Check sheet for the modelled part. Datum: model origin and axes. Units: mm. A direction names the side the tool comes from. Round coordinates to 2 decimals unless told otherwise and drop trailing zeros. Write each loop counter-clockwise with the first axis right and the second up, starting at its lowest first coordinate (ties: lowest second). Pieces come first, ordered by that corner, then holes. Notation, with made-up numbers: (-4, 24) -> (30, 24) arc R30 ccw to (30, 51) -> close; hole circle Ø10 at (46.5, 42). An arc over 180 degrees is marked (long way). One line per item, written item: value.
Autodesk Inventor part; units mm, degrees
ref_plane "Start plane" through (0, 0, -63.5) normal (0, 0, 1) x (1, 0, 0)
ref_plane "End plane" through (0, 0, 777.875) normal (0, 0, 1) x (1, 0, 0)
ref_plane "Work Plane3" through (0, -454.025, -63.5) normal (0, 0, -1) x (-1, 0, 0)
ref_plane "Start plane" through (0, 0, -63.5) normal (0, 0, 1) x (1, 0, 0)
ref_plane "End plane" through (0, 0, 777.875) normal (0, 0, 1) x (1, 0, 0)
sketch "Sketch" plane through (0, 0, 0) normal (0, 0, 1) x (1, 0, 0)
  line L0 (63.5, 0) -> (0, 0)
  line L1 (0, 0) -> (0, 63.5)
  line L2 (0, 63.5) -> (0.9525, 63.5)
  line L3 (4.7625, 59.69) -> (4.7625, 12.6365)
  line L4 (12.6365, 4.7625) -> (59.69, 4.7625)
  line L5 (63.5, 0.9525) -> (63.5, 0)
  line L6 (0, -11.0414) -> (0, 31.5385) construction
  line L7 (-11.0414, 0) -> (31.5385, 0) construction
  arc A0 (4.7625, 12.6365) -> (12.6365, 4.7625) centre (12.6365, 12.6365) ccw
  arc A1 (4.7625, 59.69) -> (0.9525, 63.5) centre (0.9525, 59.69) ccw
  arc A2 (63.5, 0.9525) -> (59.69, 4.7625) centre (59.69, 0.9525) ccw
  line L8 (0, 79.3552) -> (0, -26.1075) construction
  line L9 (-26.1075, 0) -> (79.3552, 0) construction
  point P0 (4.7625, 63.5)
  point P1 (4.7625, 4.7625)
  point P2 (63.5, 4.7625)
  dimension "d0" = 63.5
  dimension "d1" = 63.5
  dimension "d2" = 4.7625
  dimension "d3" = 4.7625
  dimension "d10" = 0
  dimension "d11" = 0
  dimension "d14" = 7.874
  dimension "d15" = 3.81
extrude "Body" add sketch "Sketch" along normal up to surface (841.375 mm away) from surface at -63.5
sketch "Sketch3" plane through (0, 0, 0) normal (0, 0, 1) x (1, 0, 0)
  line L0 (0, 0) -> (10, 0)
ref_plane "Work Plane4" through (0, 0, 0) normal (0, -1, 0) x (1, 0, 0)
sketch "Sketch4" plane through (0, 0, 0) normal (0, -1, 0) x (1, 0, 0)
  line L0 (-2, -63.5) -> (12, -63.5)
  line L1 (-2, 777.875) -> (12, 777.875)
  dimension "d17" = 841.375
ref_plane "Work Plane3" through (0, -454.025, -63.5) normal (0, 0, -1) x (-1, 0, 0)
split "Split1" plane through (0, -454.025, -63.5) removes the side toward (0, 0, -1)
equation "\"d0\" = G_H"
equation "\"d1\" = G_H"
equation "\"d2\" = G_T"
equation "\"d3\" = G_T"
equation "\"d14\" = G_IR"
equation "\"d15\" = G_ER"
equation "\"d4\" = G_L"
equation "\"G_H\" = 63.5"
equation "\"G_T\" = 4.7625"
equation "\"G_ER\" = 3.81"
equation "\"G_IR\" = 7.874"
equation "\"G_L\" = d17"
equation "\"ex\" = 0"
equation "\"G_OFFSET_START\" = 63.5"
equation "\"G_OFFSET_END\" = 0"
equation "\"d12\" = -G_OFFSET_START"
equation "\"d13\" = G_OFFSET_END + B_L"
equation "\"B_L\" = 777.875"
properties part number "ANSI L 2.5 x 2.5 x 3_16 00000003"
Item 1: Thickness scan on line 1 (X direction, y = 25, z = 150); line 2 (X direction, y = 60.5, z = 454). Record the ranges inside material, lowest first.
Answer:
line 1: x = 0 to 4.76
line 2: x = 0 to 4.68
Item 2: Sectioned sample at A-A on z = 512. Enter the section's corners in (x, y), and give its area (3 significant figures).
Answer:
outline: (0, 0) -> (63.5, 0) -> (63.5, 0.95) arc R3.81 ccw to (59.69, 4.76) -> (12.64, 4.76) arc R7.87 cw to (4.76, 12.64) -> (4.76, 59.69) arc R3.81 ccw to (0.95, 63.5) -> (0, 63.5) -> close
area: 589 mm^2
Item 3: Sectioned sample at B-B on x = 51. Enter the section's corners in (y, z) (1 decimal).
Answer:
outline: (0, -63.5) -> (4.8, -63.5) -> (4.8, 777.9) -> (0, 777.9) -> close
Item 4: Tool access check on faces 1 (the flat face through (36, 4.762, 351)), 2 (the flat face through (32, 0, 351)). Record the directions out of +Z, -Z, +X, -X, +Y, -Y that give a thin tool (end or side, any length) a straight path to the whole face; none if there is none.
Answer:
face 1: +Z, -Z, +X, +Y
face 2: +Z, -Z, +X, -X, -Y
Item 5: Depth check by flat-ended pin: P1, Ø14, axis at x = 29.5, z = 264.5, coming from the +Y side; P2, Ø12, axis at x = 52.5, y = 11.5, coming from the -Z side; P3, Ø4, axis at y = 17, z = 286.5, coming from the -X side; P4, Ø14, axis at y = 34.5, z = 429, coming from the +X side. Enter the tip coordinate at first touch or a pass-through.
Answer:
P1: stops at y = 4.76
P2: passes through
P3: stops at x = 0
P4: stops at x = 4.76
